Input: part model. Units: mm. Frame: model coordinates. Round coordinates to 2 decimals unless told otherwise and drop trailing zeros. Answer as a JSON object with one key per item and string values. Group by question number.
Item 1: Pin query (flat end, axial travel): pin 1 (1 mm diameter, centred on x = 3.5, y = -2.5, fed in from +Z); pin 2 (1.7 mm diameter, centred on y = -2.78, z = 41.96, fed in from -X). Return the tip coordinate at first contact, or that it passes through.
Item 2: Material intervals for line 1 (Z direction, x = -2, y = -3); line 2 (Z direction, x = 0.75, y = -3.5); line 3 (Z direction, x = 1, y = -1), sorted ascending. Write a range as [from, to].
Item 3: Draft query along Y for faces 1 (the cylindrical face through (0.156, -2.963, 43.347)), 2 (the flat face through (0, -6.35, 1)), 3 (the flat face through (-11.176, -3, -1)). Return one class per face: released by +Y, released by -Y, zero draft, split by the parting line, or undercut.
from build123d import *

# Parameters (mm, degrees)
F0_W          = 22.352
F0_H          = 88.9
F1_DEPTH      = 6.35
F2_R          = 1.397
F3_DEPTH      = 15.24
F3_DEPTH_BACK = 15.24
F4_R          = 3.188693


with BuildPart() as f1:
    # F0 (on Front) → F1 (new body)
    with BuildSketch(Plane.XZ):
        Rectangle(F0_W, F0_H)
    extrude(amount=F1_DEPTH)

    # F2 (on Right) → F3 (cut, two sides)
    with BuildSketch(Plane.YZ) as f3_sk:
        with Locations((-2.781508, 41.962247)):
            Circle(F2_R)
    extrude(amount=F3_DEPTH, mode=Mode.SUBTRACT)
    extrude(f3_sk.sketch, amount=-F3_DEPTH_BACK, mode=Mode.SUBTRACT)

    # F4
    f4_edges = [f1.edges().sort_by_distance(p)[0] for p in [
        (0, 0, 44.45),
    ]]
    fillet(f4_edges, radius=F4_R)


solid = f1.part
Solved:
{
 "1": {"pin 1": "z = 44.44", "pin 2": "through"},
 "2": {"line 1": "[-44.45, 40.58], [43.34, 44.44]", "line 2": "[-44.45, 40.76], [43.16, 44.45]", "line 3": "[-44.45, 43.58]"},
 "3": {"face 1": "undercut", "face 2": "released by -Y", "face 3": "zero draft"}
}
